The figure shows three views and two pictorial views of one solid part (mm, origin at its lowest corner). Answer the questions. A direction names the side the tool comes from. Give positions to 0.01 mm unless a question says otherwise; leave off trailing zeros. Loops run counter-clockwise (first coordinate to the right, second up) from the corner with the lowest first, then second, coordinate; pieces in that order, holes last. Notation, with made-up numbers: (28.25, -4.5) - (47.25, -4.5) arc R22 ccw to (47.25, 10.5) - close; hole circle Ø8 at (52, -16.5). An arc over 180 degrees is marked (long way). Write item = value, one per line.
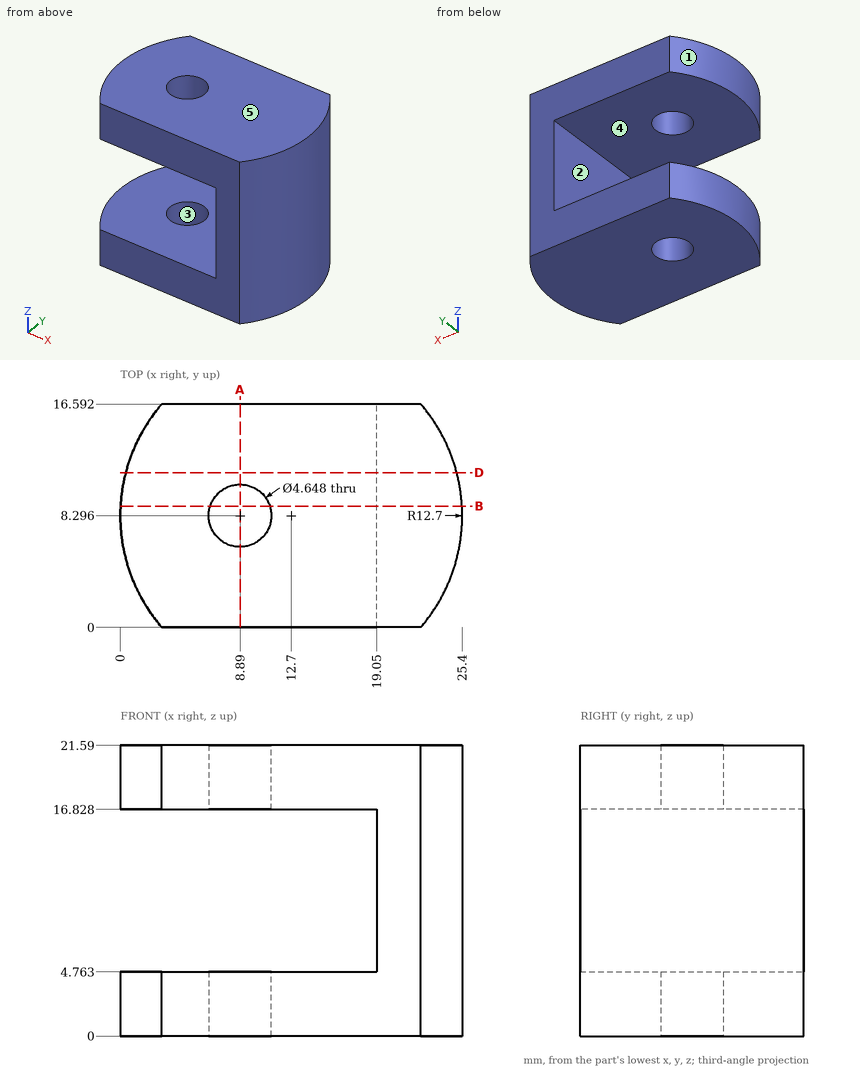
1) A tool of negligible diameter and unlimited length cuts with its end or side. For the marked faces 1 and 2, from which of +Z, -Z, +X, -X, +Y, -Y can it reach the whole face along a straight path? Write none if from no direction.
Output:
face_1 = +Z, -Z, -X
face_2 = -X, +Y, -Y
2) A cutting plane is placed at A-A on x = 8.89. Determine the outline of the cut face in (y, z), then the cut area to 3 significant figures.
Output:
outline = (0, 0) - (5.97, 0) - (5.97, 4.76) - (0, 4.76) - close; (0, 16.83) - (5.97, 16.83) - (5.97, 21.59) - (0, 21.59) - close; (10.62, 0) - (16.59, 0) - (16.59, 4.76) - (10.62, 4.76) - close; (10.62, 16.83) - (16.59, 16.83) - (16.59, 21.59) - (10.62, 21.59) - close
area = 114 mm²
3) Find the intervals of material crossed by probe 1 along Z at (x, y) = (6.75, 5.5); probe 2 along Y at (x, z) = (8.89, 3); probe 3 along Y at (x, z) = (7.5, 17.5) (1 decimal), in increasing order.
Output:
probe_1 = 0 to 4.76, 16.83 to 21.59
probe_2 = 0 to 5.97, 10.62 to 16.59
probe_3 = 0 to 6.4, 10.2 to 16.6
4) The mould has two halves that part along Z. Classify the marked faces 3, 4 and 5: pulls with the +Z half, pulls with the -Z half, needs draft (parallel to the pull), parting line crosses it, or undercut.
Output:
face_3 = needs draft
face_4 = undercut
face_5 = pulls with the +Z half
5) A cutting plane is placed at B-B on y = 9. Give the number of separate pieces and of enclosed holes in the cut face, then the cut area to 3 significant figures.
Output:
separate_pieces = 3
enclosed_holes = 0
area = 276 mm²
6) Each of these flat-tipped pins is pushed along its axis until it touches: P1, Ø4, axis at y = 12.5, z = 4.5, coming from the +X side; P2, Ø9.5, axis at y = 8.5, z = 10.5, coming from the -X side. Where does it stop, or does it pass through?
Output:
P1 = 25.21
P2 = 19.05
7) A cutting plane is placed at D-D on y = 11.5. Determine the outline of the cut face in (x, z).
Output:
outline = (0.41, 0) - (24.99, 0) - (24.99, 21.59) - (0.41, 21.59) - (0.41, 16.83) - (19.05, 16.83) - (19.05, 4.76) - (0.41, 4.76) - close
